Verification items for the finished model (mm, model axes). A direction names the side the tool comes from. Round coordinates to 2 decimals unless told otherwise and drop trailing zeros. Write each loop counter-clockwise with the first axis right and the second up, starting at its lowest first coordinate (ties: lowest second). Pieces come first, ordered by that corner, then holes. Notation, with made-up numbers: M -37.75,-21.5 L 12.25,-21.5 A22 cw 12.25,12.5 Z; hole C -3.75,15.5 d8. An arc over 180 degrees is marked long. Use a Markdown table: item, result. Add a question column.
from build123d import *

# Parameters (mm, degrees)
SKETCH_R             = 1.7
PAD_DEPTH            = 8.5
SKETCH002_R          = 3.1
POCKET_DEPTH         = 3.5
POCKET001_DEPTH      = 1
POCKET001_DEPTH_BACK = -5
SKETCH004_R          = 2.7
POCKET002_DEPTH      = 5.001
FILLET_R             = 0.5


with BuildPart() as part:
    # Sketch → Pad (new body, symmetric)
    with BuildSketch(Plane.XZ):
        Polygon((-13.9, 5), (13.9, 5), (13.9, 3.5), (16.836849, 0), (13.9, -3.5), (13.9, -5), (-13.9, -5), (-13.9, -3.5), (-16.836849, 0), (-13.9, 3.5), align=None)
        with Locations((-11, 0)):
            Circle(SKETCH_R, mode=Mode.SUBTRACT)
        with Locations((11, 0)):
            Circle(SKETCH_R, mode=Mode.SUBTRACT)
    extrude(amount=PAD_DEPTH, both=True)

    # Sketch002 (on DatumPlane) → Pocket (cut)
    with BuildSketch(Plane.XZ.offset(8.5)):
        with Locations((-11, 0)):
            Circle(SKETCH002_R)
        with Locations((11, 0)):
            Circle(SKETCH002_R)
    extrude(amount=-POCKET_DEPTH, mode=Mode.SUBTRACT)

    # Sketch003 → Pocket001 (cut, two sides)
    with BuildSketch(Plane.XY) as pocket001_sk:
        Polygon((4.25, -2.453739), (4.25, 2.453739), (0, 4.907477), (-4.25, 2.453739), (-4.25, -2.453739), (0, -4.907477), align=None)
    extrude(amount=-POCKET001_DEPTH, mode=Mode.SUBTRACT)
    extrude(pocket001_sk.sketch, amount=-POCKET001_DEPTH_BACK, mode=Mode.SUBTRACT)

    # Sketch004 → Pocket002 (cut, through all)
    with BuildSketch(Plane.XY):
        Circle(SKETCH004_R)
    extrude(amount=-POCKET002_DEPTH, mode=Mode.SUBTRACT)

    # Fillet
    fillet_edges = [part.edges().sort_by_distance(p)[0] for p in [
        (16.836849, 0, 0),
        (-16.836849, 0, 0),
    ]]
    fillet(fillet_edges, radius=FILLET_R)


solid = part.part
1. Cross-section at A-A on x = -11. Enter the section's corners in (y, z), plus the area to 3 significant figures.
2. Depth check by flat-ended pin: pin 1 Ø1.9 at (x, z) = (11.5, -0.5) entering from -Y; pin 2 Ø4 at (x, y) = (-0.5, 2) entering from +Z; pin 3 Ø0.8 at (y, z) = (-4, -4) entering from -X; pin 4 Ø1 at (y, z) = (-4, -3.5) entering from -X. Enter the tip coordinate at first touch or a pass-through.
3. Cross-section at D-D on y = 6.75. Enter the section's corners in (x, z).
4. Access from +Z, -Z, +X, -X, +Y, -Y to the whole of each face (thin tool, end or side, straight path). Record for faces 4 (the cylindrical face through (-0.585, -2.636, -2.972)), 5 (the flat face through (-2.095, 3.698, 1.958)), 6 (the flat face through (12.33, -5, -1.33)).
5. Release check for a two-part mould opening along Z. For faces 1 (the flat face through (-3, -4, 5)), 2 (the flat face through (13.9, 0, 4)), 3 (the cylindrical face through (12.57, 1.84, -0.65)) record: +Z half, -Z half, draft (parallel to the pull), parting line (faces both ways), or undercut.
6. Cross-section at B-B on y = 0. Enter the section's corners in (x, z).
7. Scan lines: line 1 along Z through (x, y) = (-11, -6.35); line 2 along X through (y, z) = (-7.25, -0.25); line 3 along X through (y, z) = (7.75, 0.5). Record each from-to range of solid material in increasing order. Write a range as from..to.
8. Cross-section at C-C on z = 0.75. Enter the section's corners in (x, y).
Answer:
| question | item | result |
|---|---|---|
| 1 | outline | M -8.5,-5 L 8.5,-5 L 8.5,-1.7 L -5,-1.7 L -5,-3.1 L -8.5,-3.1 Z; M -8.5,3.1 L -5,3.1 L -5,1.7 L 8.5,1.7 L 8.5,5 L -8.5,5 Z |
| 1 | area | 102 mm^2 |
| 2 | pin 1 | passes through |
| 2 | pin 2 | stops at z = -1 |
| 2 | pin 3 | stops at x = -13.9 |
| 2 | pin 4 | stops at x = -14.32 |
| 3 | outline | M -16.57,-0.32 L -13.9,-3.5 L -13.9,-5 L 13.9,-5 L 13.9,-3.5 L 16.57,-0.32 A0.5 ccw 16.57,0.32 L 13.9,3.5 L 13.9,5 L -13.9,5 L -13.9,3.5 L -16.57,0.32 A0.5 ccw Z; hole C -11,0 d3.4; hole C 11,0 d3.4 |
| 4 | face 4 | +Z, -Z |
| 4 | face 5 | +Z |
| 4 | face 6 | -Y |
| 5 | face 1 | +Z half |
| 5 | face 2 | draft |
| 5 | face 3 | undercut |
| 6 | outline | M -16.57,-0.32 L -13.9,-3.5 L -13.9,-5 L -2.7,-5 L -2.7,-1 L -4.25,-1 L -4.25,5 L -13.9,5 L -13.9,3.5 L -16.57,0.32 A0.5 ccw Z; M 2.7,-5 L 13.9,-5 L 13.9,-3.5 L 16.57,-0.32 A0.5 ccw 16.57,0.32 L 13.9,3.5 L 13.9,5 L 4.25,5 L 4.25,-1 L 2.7,-1 Z; hole C -11,0 d3.4; hole C 11,0 d3.4 |
| 7 | line 1 | z = -5..-3.1, 3.1..5 |
| 7 | line 2 | x = -16.62..-14.09, -7.91..7.91, 14.09..16.62 |
| 7 | line 3 | x = -16.42..-12.62, -9.38..9.38, 12.62..16.42 |
| 8 | outline | M -16.21,-8.5 L -14.01,-8.5 L -14.01,-5 L -12.53,-5 L -12.53,8.5 L -16.21,8.5 Z; M -9.47,-5 L -7.99,-5 L -7.99,-8.5 L 7.99,-8.5 L 7.99,-5 L 9.47,-5 L 9.47,8.5 L -9.47,8.5 Z; M 12.53,-5 L 14.01,-5 L 14.01,-8.5 L 16.21,-8.5 L 16.21,8.5 L 12.53,8.5 Z; hole M -4.25,-2.45 L 0,-4.91 L 4.25,-2.45 L 4.25,2.45 L 0,4.91 L -4.25,2.45 Z |
